Design review of the part built by this model. Coordinates are the model's own, in mm. Round coordinates to 2 decimals unless told otherwise and drop trailing zeros. Loops run counter-clockwise (first coordinate to the right, second up) from the corner with the lowest first, then second, coordinate; pieces in that order, holes last. Notation, with made-up numbers: M 65.25,5 L 71.25,5 A11 ccw 71.25,25 Z; hole C 42,89.5 d1. An arc over 180 degrees is marked long. One line per item, written item: value. Start each with the question number.
Item 1: Mouldability with a two-part tool opening along X and no side actions: class faces 1 (the flat face through (2, 2, 0.7)), 2 (the cylindrical face through (-0.54, -2.44, 3.31)) as released by +X, released by -X, zero draft, split by the parting line, or undercut.
Item 2: We need section A-A (x = 0). Write out the cut boundary in (y, z), then the cut area to 3 significant figures.
Item 3: Clearance check with flat-ended pins moving along their axes: pin 1 (3 mm diameter, centred on x = 2, y = -2.5, fed in from -Z); pin 2 (0.5 mm diameter, centred on y = 0, z = -1.5, fed in from -X); pin 3 (0.5 mm diameter, centred on x = 1, z = -1.5, fed in from -Y). State where each tip first meets the part, or that it passes through.
Item 4: We need section D-D (x = 1.35). Write out the cut boundary in (y, z), then the cut area to 3 significant figures.
Item 5: We need section C-C (z = 2.25). Write out the cut boundary in (x, y), then the cut area to 3 significant figures.
Item 6: We need section B-B (y = 2.1). Write out the cut boundary in (x, z).
Item 7: For line 1 along Z through (x, y) = (-2.15, -1.7); line 2 along X through (y, z) = (0.15, 8); line 3 along X through (y, z) = (-0.95, 2.75), list the stretches that pass through material, from the lowest coordinate up.
from build123d import *

# Parameters (mm, degrees)
F0_R     = 2.5
F1_DEPTH = 6
F5_DEPTH = 0.7
F6_W     = 0.6
F6_H     = 0.6
F7_DEPTH = 3


with BuildPart() as f1:
    # F0 (on Top) → F1 (new body)
    with BuildSketch(Plane.XY):
        Circle(F0_R)
    extrude(amount=F1_DEPTH)

    # F2 (on face) → F3 (revolve)
    with BuildSketch(Plane.XY.offset(6)):
        with BuildLine():
            ThreePointArc((0, 2.5), (-2.5, 0), (0, -2.5))
            Line((0, -2.5), (0, 2.5))
        make_face()
    revolve(axis=Axis((0, 0, 6), (0, 1, 0)))

    # F4 (on face) → F5 (join)
    with BuildSketch(Plane(origin=(0, 0, 0), x_dir=(1, 0, 0), z_dir=(0, 0, -1))):
        with BuildLine():
            Line((-2.5, 1.658312), (-2.5, -1.658312))
            ThreePointArc((-2.5, -1.658312), (3, 0), (-2.5, 1.658312))
        make_face()
    extrude(amount=-F5_DEPTH)

    # F6 (on face) → F7 (join)
    with BuildSketch(Plane(origin=(0, 0, 0), x_dir=(1, 0, 0), z_dir=(0, 0, -1))):
        with Locations((1.25, 0)):
            Rectangle(F6_W, F6_H)
        with Locations((-1.25, 0)):
            Rectangle(F6_W, F6_H)
    extrude(amount=F7_DEPTH)


solid = f1.part
A:
1. face 1: zero draft
1. face 2: split by the parting line
2. outline: M -3,0 L 3,0 L 3,0.7 L 2.5,0.7 L 2.5,6 A2.5 ccw -2.5,6 L -2.5,0.7 L -3,0.7 Z
2. area: 40.5 mm2
3. pin 1: z = 0
3. pin 2: x = -1.55
3. pin 3: y = -0.3
4. outline: M -2.68,0 L -0.3,0 L -0.3,-3 L 0.3,-3 L 0.3,0 L 2.68,0 L 2.68,0.7 L 2.1,0.7 L 2.1,6 A2.1 ccw -2.1,6 L -2.1,0.7 L -2.68,0.7 Z
4. area: 34.8 mm2
5. outline: C 0,0 d5
5. area: 19.6 mm2
6. outline: M -2.14,0 L 2.14,0 L 2.14,0.7 L 1.36,0.7 L 1.36,6 A1.36 ccw -1.36,6 L -1.36,0.7 L -2.14,0.7 Z
7. line 1: 0 to 0.7
7. line 2: -1.49 to 1.49
7. line 3: -2.31 to 2.31
